from build123d import *

# Parameters (mm, degrees)
F1_DEPTH       = 42
F1_DEPTH_BACK  = 42
F3_DEPTH       = 3
F4_W           = 171.0703811337
F4_H           = 30
F5_DEPTH       = 31.501
F6_R           = 5
F8_D           = 5
F8_CSINK_D     = 10
F8_CSINK_ANGLE = 90


# Not quite as in the source:
# - a pattern or mirror of a feature is missing from the dataset's text; its kind, count and spacing are read off the source's solid


with BuildPart() as f1:
    # F0 (on Front) → F1 (new body, two sides)
    with BuildSketch(Plane.XZ) as f1_sk:
        with BuildLine():
            Line((-74.8302465006, 17.25), (-74.8302465006, 14.25))
            Line((-74.8302465006, 14.25), (20.1697534994, 14.25))
            ThreePointArc((20.1697534994, 14.25), (34.429081055, 0.4973529093), (21.2011066634, -14.25))
            Line((21.2011066634, -14.25), (-104.8302465006, -14.25))
            Line((-104.8302465006, -14.25), (-104.8302465006, -17.25))
            Line((-104.8302465006, -17.25), (21.3044886882, -17.25))
            ThreePointArc((21.3044886882, -17.25), (37.4290815856, 0.5490131867), (20.1697534994, 17.25))
            Line((20.1697534994, 17.25), (-74.8302465006, 17.25))
        make_face()
    extrude(amount=F1_DEPTH)
    extrude(f1_sk.sketch, amount=-F1_DEPTH_BACK)

    # F2 (on face) → F3 (join)
    with BuildSketch(Plane.XZ.offset(42)):
        with BuildLine():
            Line((20.1697534994, 17.25), (-74.8302465006, 17.25))
            Line((-74.8302465006, 17.25), (-74.8302465006, -17.25))
            Line((-74.8302465006, -17.25), (21.3044886882, -17.25))
            ThreePointArc((21.3044886882, -17.25), (37.4290815856, 0.5490131867), (20.1697534994, 17.25))
        make_face()
    f3 = extrude(amount=-F3_DEPTH)

    # F3_copies: F3 across plane
    add(f3.mirror(Plane.ZX))

    # F4 (on face) → F5 (cut, through all)
    with BuildSketch(Plane.XY.offset(-14.25)):
        with Locations((-19.9944982305, 0)):
            Rectangle(F4_W, F4_H)
    extrude(amount=F5_DEPTH, mode=Mode.SUBTRACT)

    # F6
    f6_edges = [f1.edges().sort_by_distance(p)[0] for p in [
        (-104.830247, -42, -15.75),
        (-104.830247, 42, -15.75),
    ]]
    fillet(f6_edges, radius=F6_R)

    # F8 (through all)
    with Locations(Plane.XY.offset(-14.25)):
        with Locations((-89.8302465006, -16.0900652409), (-89.8302465006, 16.0900652409), (0, 0)):
            CounterSinkHole(F8_D / 2, F8_CSINK_D / 2, counter_sink_angle=F8_CSINK_ANGLE)


solid = f1.part
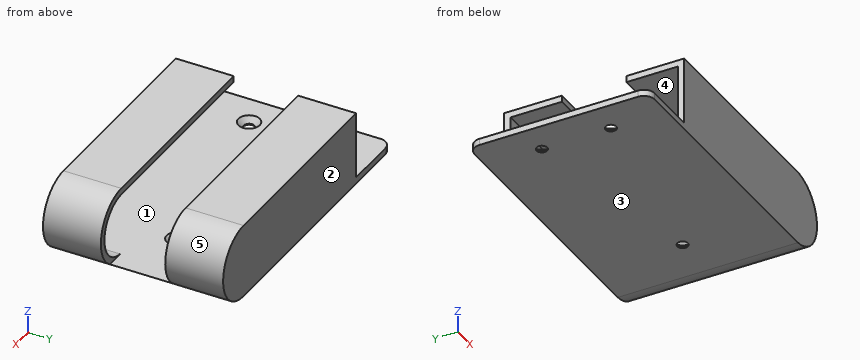
Input: part model. Units: mm. Frame: model coordinates. Face numbers are marked on the shaded views. A direction names the side the tool comes from. Coordinates: 2 decimals unless noted, no trailing zeros. Loops run counter-clockwise (first coordinate to the right, second up) from the corner with the lowest first, then second, coordinate; pieces in that order, holes last.
Q1. Cut plane C-C (x = 0). Output: boundary loops of the cut face in (y, z).
Q2. Contact query for flat-ended pins moving along their axis: pin 1 (8 mm diameter, centred on x = -89.83, y = -16.09, fed in from -Z); pin 2 (4.5 mm diameter, centred on x = -89.83, y = 16.09, fed in from +Z); pin 3 (4 mm diameter, centred on x = -82.5, y = 3, fed in from +Z); pin 4 (5 mm diameter, centred on y = -18.5, z = -8, fed in from -X). Output: stop coordinate, or through.
Q3. Draft query along Y for the marked faces 1, 2 and 3. Return one class per face: +Y half, -Y half, draft (parallel to the pull), parting line (faces both ways), or undercut.
Q4. Cut plane D-D (x = -70.5). Output: boundary loops of the cut face in (y, z).
Q5. Cut plane A-A (y = 0). Output: boundary loops of the cut face in (x, z), then the cut area to 3 significant figures.
Q6. Set-up query: the marked faces 4 and 5. Return all of +Z, -Z, +X, -X, +Y, -Y with unobstructed straight access to the full face (end or side cutting, diameter ignored); none if empty.
Q7. Material intervals for line 1 (Y direction, x = -6, z = -13.5); line 2 (Z direction, x = -16, y = -22); line 3 (Y direction, x = 0, z = -17), sorted ascending.
Q8. Cut plane B-B (z = 10). Output: boundary loops of the cut face in (x, y), then the cut area to 3 significant figures.
Working result:
1. outline: (-42, -17.25) - (-2.5, -17.25) - (-2.5, -16.75) - (-5, -14.25) - (-39, -14.25) - (-39, 14.25) - (-15, 14.25) - (-15, 17.25) - (-42, 17.25) - close; (2.5, -17.25) - (42, -17.25) - (42, 17.25) - (15, 17.25) - (15, 14.25) - (39, 14.25) - (39, -14.25) - (5, -14.25) - (2.5, -16.75) - close
2. pin 1: stops at z = -17.25
2. pin 2: passes through
2. pin 3: stops at z = -14.25
2. pin 4: stops at x = 29.85
3. face 1: undercut
3. face 2: +Y half
3. face 3: draft
4. outline: (-42, -17.25) - (42, -17.25) - (42, 17.25) - (15, 17.25) - (15, 14.25) - (39, 14.25) - (39, -14.25) - (-39, -14.25) - (-39, 14.25) - (-15, 14.25) - (-15, 17.25) - (-42, 17.25) - close
5. outline: (-104.83, -17.25) - (-2.5, -17.25) - (-2.5, -16.75) - (-5, -14.25) - (-104.83, -14.25) - close; (2.5, -17.25) - (21.3, -17.25) arc R17.27 ccw to (29.95, -14.25) - (5, -14.25) - (2.5, -16.75) - close
5. area: 374 mm2
6. face 4: -X
6. face 5: +X, +Y, -Y
7. line 1: y = -42 to -39, 39 to 42
7. line 2: z = -17.25 to -14.25, 14.25 to 17.25
7. line 3: y = -42 to -2.5, 2.5 to 42
8. outline: (-74.83, -42) - (34.24, -42) - (34.24, -15) - (30.33, -15) - (30.33, -39) - (-74.83, -39) - close; (-74.83, 39) - (30.33, 39) - (30.33, 15) - (34.24, 15) - (34.24, 42) - (-74.83, 42) - close
8. area: 842 mm2
